Could you check a few things on this model? Use its own coordinates, in mm. A direction names the side the tool comes from. Round coordinates to 2 decimals unless told otherwise and drop trailing zeros. Order: outer loops, then holes, each group sorted by start corner. A loop starts at its lowest first (then second) coordinate and runs counter-clockwise, first axis right, second up. Notation, with made-up numbers: M -9.75,60 L 26.25,60 A11 cw 26.25,73 Z; hole C 9,20.25 d10. An arc over 180 degrees is marked long. Write each question's results on one line, items separated by ' | '. Start each with the question number.
1. Suppose I cut it at B-B on x = -101. Write out the boundary of the cut face in (y, z).
2. Suppose I cut it at A-A on x = -29. Give the number of separate pieces and of enclosed holes in the cut face, and give its area (3 significant figures).
3. Please list where these lines run through material, in increasing order: L1, parallel to Y at x = 102.5, z = 85.5; L2, parallel to Z at x = -6, y = -35; L3, parallel to Z at x = -76, y = -126.
4. We'd pull the mould along Z, two halves only. Please class faces 1 (the cylindrical face through (238.868, 87.596, 128.102)), 2 (the flat face through (167, 3, 251.46)), 3 (the flat face through (258.572, 73, 51)): released by +Z, released by -Z, zero draft, split by the parting line, or undercut.
5. I'm going to push flat-ended pins straight in: pin 1 (4 mm diameter, centred on x = 92, y = -71, fed in from +Z); pin 2 (4 mm diameter, centred on x = 23.5, z = 155, fed in from -Y); pin 3 (2 mm diameter, centred on y = -35, z = 252.5, fed in from +X). Where does each tip first touch, or does it pass through?
6. For faces 4 (the flat face through (176.072, -3, 233)), 5 (the flat face through (-93, -69.375, 212)), 6 (the flat face through (157.62, 3, 233)), 7 (the flat face through (-44.997, -99.9, 121.4)), 8 (the flat face through (40, -124, 215.9)), which set-ups out of +Z, -Z, +X, -X, +Y, -Y let a thin tool reach every point of the face, with its end or its side?
from build123d import *

# Parameters (mm, degrees)
F0_W      = 154.8604735136
F0_H      = 381
F0_W_2    = 202.8337074444
F0_W_3    = 150.305819042
F1_DEPTH  = 215.9
F3_DEPTH  = 365.76
F4_DEPTH  = 474.472
F5_DEPTH  = 384.81
F6_DEPTH  = 463.296
F7_DEPTH  = 453.644
F8_DEPTH  = 401.828
F9_W      = 333.3268084526
F9_H      = 308.1617667079
F10_DEPTH = 101.6
F12_DEPTH = 332.74
F13_DEPTH = 290.83
F14_W     = 640.7658
F14_H     = 381.7952661514
F15_DEPTH = 7.62
F16_W     = 18.4519021228
F16_H     = 174.1818501353
F16_H_2   = 32.6362997293
F17_DEPTH = 35.56
F18_R     = 44.8167953051
F18_R_2   = 38.1
F19_DEPTH = 258.572
F20_DEPTH = 485.14
F21_DEPTH = 258.572
F22_DEPTH = 57.658
F23_DEPTH = 72.898
F24_DEPTH = 250.19
F25_W     = 142.1934430047
F25_H     = 97.1279808664
F26_DEPTH = 68.58
F28_DEPTH = 340.868
F30_W     = 177.6428297162
F30_H     = 182.6925156638
F31_DEPTH = 723.9


# Not quite as in the source:
# - the program builds the solid bodies; features that only make, move or delete a surface that nothing else refers to are left out


with BuildPart() as f1:
    # F0 (on Top) → F1 (new body)
    with BuildSketch(Plane.XY):
        with Locations((-176.5697632432, 0)):
            Rectangle(F0_W, F0_H)
        with Locations((2.2773272358, 0)):
            Rectangle(F0_W_2, F0_H)
        with Locations((178.847090479, 0)):
            Rectangle(F0_W_3, F0_H)
    extrude(amount=F1_DEPTH)

    # F2 (on face) → F3 (cut)
    with BuildSketch(Plane.XZ.offset(190.5)):
        Polygon((-244.8522895575, 194.3728802726), (-244.8522895575, 10.3632332757), (244.8522895575, 10.3632332757), (175.2408137327, 194.3728802726), align=None)
    extrude(amount=-F3_DEPTH, mode=Mode.SUBTRACT)

    # F2 (on face) → F4 (cut)
    with BuildSketch(Plane.XZ.offset(190.5)):
        Polygon((215.0387168483, 194.3728802726), (244.8522895575, 115.5642510209), (244.8522895575, 194.3728802726), align=None)
    extrude(amount=-F4_DEPTH, mode=Mode.SUBTRACT)

    # F2 (on face) → F5 (cut)
    with BuildSketch(Plane.XZ.offset(190.5)):
        Polygon((244.8522895575, 194.3728802726), (244.8522895575, 115.5642510209), (254, 91.3833677769), (254, 215.9), (206.8949341774, 215.9), (215.0387168483, 194.3728802726), align=None)
    extrude(amount=-F5_DEPTH, mode=Mode.SUBTRACT)

    # F2 (on face) → F6 (cut)
    with BuildSketch(Plane.XZ.offset(190.5)):
        Polygon((184.2154591353, 194.3728802726), (244.8522895575, 34.0866396952), (244.8522895575, 115.5642510209), (215.0387168483, 194.3728802726), align=None)
    extrude(amount=-F6_DEPTH, mode=Mode.SUBTRACT)

    # F2 (on face) → F7 (cut)
    with BuildSketch(Plane.XZ.offset(190.5)):
        Polygon((244.8522895575, 115.5642510209), (244.8522895575, 34.0866396952), (254, 9.9057564512), (254, 91.3833677769), align=None)
    extrude(amount=-F7_DEPTH, mode=Mode.SUBTRACT)

    # F2 (on face) → F8 (cut)
    with BuildSketch(Plane.XZ.offset(190.5)):
        Polygon((176.0716764644, 215.9), (184.2154591353, 194.3728802726), (215.0387168483, 194.3728802726), (206.8949341774, 215.9), align=None)
    extrude(amount=-F8_DEPTH, mode=Mode.SUBTRACT)

    # F9 (on face) → F10 (join)
    with BuildSketch(Plane.XY.offset(215.9)):
        with Locations((-87.3365957737, 36.4191166461)):
            Rectangle(F9_W, F9_H)
    extrude(amount=F10_DEPTH)

    # F11 (on face) → F12 (cut)
    with BuildSketch(Plane.XZ.offset(117.6617667079)):
        Polygon((62.1921845761, 266.8175234586), (79.3268084526, 266.7), (79.3268084526, 317.5), (20.0025010854, 317.5), (24.5608866934, 309.6932172775), (62.1921845761, 309.6932172775), align=None)
        Polygon((62.1921845761, 245.2451009057), (79.3268084526, 215.9), (79.3268084526, 266.7), (62.1921845761, 266.8175234586), align=None)
        Polygon((24.5608866934, 309.6932172775), (49.5453838887, 266.9042657045), (62.1921845761, 266.8175234586), (62.1921845761, 309.6932172775), align=None)
        Polygon((49.5453838887, 266.9042657045), (62.1921845761, 245.2451009057), (62.1921845761, 266.8175234586), align=None)
    extrude(amount=-F12_DEPTH, mode=Mode.SUBTRACT)

    # F11 (on face) → F13 (cut)
    with BuildSketch(Plane.XZ.offset(117.6617667079)):
        Polygon((-87.3365957737, 267.843115824), (39.5991766547, 266.9724850411), (14.6545127754, 309.6932172775), (-87.3365957737, 309.6932172775), align=None)
        Polygon((-244.3442642689, 268.9200046058), (-87.3365957737, 267.843115824), (-87.3365957737, 309.6932172775), (-244.3442642689, 309.6932172775), align=None)
        Polygon((-87.3365957737, 228.2792460185), (62.1921845761, 228.2792460185), (39.5991766547, 266.9724850411), (-87.3365957737, 267.843115824), align=None)
        Polygon((-244.3442642689, 228.2792460185), (-87.3365957737, 228.2792460185), (-87.3365957737, 267.843115824), (-244.3442642689, 268.9200046058), align=None)
    extrude(amount=-F13_DEPTH, mode=Mode.SUBTRACT)

    # F14 (on face) → F15 (join)
    with BuildSketch(Plane(origin=(0, 0, 0), x_dir=(1, 0, 0), z_dir=(0, 0, -1))):
        with Locations((66.3829, -0.3976330757)):
            Rectangle(F14_W, F14_H)
    extrude(amount=F15_DEPTH)

    # F16 (on face) → F17 (join)
    with BuildSketch(Plane.XY.offset(215.9)):
        with Locations((166.845725403, 103.4090749323)):
            Rectangle(F16_W, F16_H)
        with Locations((166.845725403, 0)):
            Rectangle(F16_W, F16_H_2)
        with Locations((166.845725403, -103.4090749323)):
            Rectangle(F16_W, F16_H)
    extrude(amount=F17_DEPTH)

    # F18 (on Right) → F19 (join)
    with BuildSketch(Plane.YZ):
        with Locations((-93.4298427632, 83.6668761742)):
            Circle(F18_R)
        with Locations((-93.4298427632, 83.6668761742)):
            Circle(F18_R_2, mode=Mode.SUBTRACT)
    extrude(amount=F19_DEPTH)

    # F18 (on Right) → F20 (cut)
    with BuildSketch(Plane.YZ):
        with Locations((-93.4298427632, 83.6668761742)):
            Circle(F18_R_2)
    extrude(amount=F20_DEPTH, mode=Mode.SUBTRACT)

    # F18 (on Right) → F21 (join)
    with BuildSketch(Plane.YZ):
        with Locations((93.4298427632, 83.6668761742)):
            Circle(F18_R)
        with Locations((93.4298427632, 83.6668761742)):
            Circle(F18_R_2, mode=Mode.SUBTRACT)
        with Locations((-93.4298427632, 83.6668761742)):
            Circle(F18_R)
        with Locations((-93.4298427632, 83.6668761742)):
            Circle(F18_R_2, mode=Mode.SUBTRACT)
    extrude(amount=F21_DEPTH)

    # F18 (on Right) → F22 (cut)
    with BuildSketch(Plane.YZ):
        with Locations((-93.4298427632, 83.6668761742)):
            Circle(F18_R)
        with Locations((-93.4298427632, 83.6668761742)):
            Circle(F18_R_2, mode=Mode.SUBTRACT)
        with Locations((93.4298427632, 83.6668761742)):
            Circle(F18_R)
        with Locations((93.4298427632, 83.6668761742)):
            Circle(F18_R_2, mode=Mode.SUBTRACT)
    extrude(amount=-F22_DEPTH, mode=Mode.SUBTRACT)

    # F18 (on Right) + F21_face (on face) → F23 (cut)
    with BuildSketch(Plane.YZ):
        with Locations((-93.4298427632, 83.6668761742)):
            Circle(F18_R)
        with Locations((-93.4298427632, 83.6668761742)):
            Circle(F18_R_2, mode=Mode.SUBTRACT)
        with Locations((93.4298427632, 83.6668761742)):
            Circle(F18_R)
        with Locations((93.4298427632, 83.6668761742)):
            Circle(F18_R_2, mode=Mode.SUBTRACT)
    with BuildSketch(Plane(origin=(226.0959173271, 93.4298427632, 83.6668761742), x_dir=(0, 1, 0), z_dir=(0.9353094659, 0, 0.3538307547))):
        with BuildLine():
            add(Edge.make_bspline(
                [(38.1, 0), (38.1, -70.5554024353), (-19.05, -35.2777012177), (-76.2, 0), (-19.05, 35.2777012177), (38.1, 70.5554024353), (38.1, 0)],
                knots=[1.5707963268, 1.5707963268, 1.5707963268, 3.6651914292, 3.6651914292, 5.7595865316, 5.7595865316, 7.853981634, 7.853981634, 7.853981634], degree=2, weights=[1, 0.5, 1, 0.5, 1, 0.5, 1]))
        make_face()
    extrude(amount=-F23_DEPTH, dir=(1, 0, 0), mode=Mode.SUBTRACT)

    # F18 (on Right) → F24 (join)
    with BuildSketch(Plane.YZ):
        with Locations((-93.4298427632, 83.6668761742)):
            Circle(F18_R)
        with Locations((-93.4298427632, 83.6668761742)):
            Circle(F18_R_2, mode=Mode.SUBTRACT)
        with Locations((93.4298427632, 83.6668761742)):
            Circle(F18_R)
        with Locations((93.4298427632, 83.6668761742)):
            Circle(F18_R_2, mode=Mode.SUBTRACT)
    extrude(amount=-F24_DEPTH)

    # F25 (on face) → F26 (cut)
    with BuildSketch(Plane.XY.offset(228.2792460185)):
        with Locations((-162.1727613487, -20.8107571411)):
            Rectangle(F25_W, F25_H)
        with Locations((-19.979318344, -20.8107571411)):
            Rectangle(F25_W, F25_H)
        with Locations((-162.1727613487, 76.3172237253)):
            Rectangle(F25_W, F25_H)
        with Locations((-19.979318344, 76.3172237253)):
            Rectangle(F25_W, F25_H)
    extrude(amount=-F26_DEPTH, mode=Mode.SUBTRACT)

    # F27 (on face) → F28 (cut)
    with BuildSketch(Plane.XZ.offset(-175.26)):
        Polygon((-44.9973344803, 128.3188015223), (-44.9973344803, 85.9577953815), (79.164236784, 85.9577953815), (79.164236784, 121.7455416918), (79.164236784, 128.3188015223), align=None)
    extrude(amount=F28_DEPTH, mode=Mode.SUBTRACT)

    # F30 (on face) → F31 (cut)
    with BuildSketch(Plane.XZ.offset(-175.26)):
        with Locations((-180.61241135, 101.7094911076)):
            Rectangle(F30_W, F30_H)
    extrude(amount=F31_DEPTH, mode=Mode.SUBTRACT)


solid = f1.part
Filled sheet:
1) outline: M -190.5,-7.62 L 191.3,-7.62 L 191.3,0 L 190.5,0 L 190.5,317.5 L -117.66,317.5 L -117.66,309.69 L 173.17,309.69 L 173.17,228.28 L 124.88,228.28 L 124.88,194.37 L 175.26,194.37 L 175.26,10.36 L -190.5,10.36 Z; M -190.5,194.37 L -69.37,194.37 L -69.37,228.28 L -117.66,228.28 L -117.66,215.9 L -190.5,215.9 Z
2) separate pieces: 6 | enclosed holes: 0 | area: 20,700 mm^2
3) L1: y = -138.21 to -131.49, -55.37 to -48.65, 48.65 to 55.37, 131.49 to 138.21, 175.26 to 190.5 | L2: z = -7.62 to 10.36, 309.69 to 317.5 | L3: z = -7.62 to 10.36, 52.88 to 63.9, 103.44 to 114.45, 194.37 to 215.9
4) face 1: undercut | face 2: released by +Z | face 3: zero draft
5) pin 1: stops at z = 215.9 | pin 2: stops at y = 175.26 | pin 3: stops at x = 58.54
6) face 4: +Z, +X, +Y, -Y | face 5: none | face 6: +Z, +Y, -Y | face 7: -Y | face 8: +Z, -Y
